The model under review builds one solid part; all positions refer to its coordinate system, in mm. Face numbers are marked on the shaded views. Coordinates: 2 decimals unless noted, no trailing zeros. Write each loop counter-clockwise with the first axis right and the second up, starting at its lowest first coordinate (ties: lowest second). Pieces come first, ordered by that corner, then holes. Notation, with made-up numbers: (40.5, 55) - (90.5, 55) arc R7 ccw to (90.5, 62) - close; hole circle Ø3 at (58.5, 31). An arc over 180 degrees is marked (long way). Put each result on its own line as item: value.
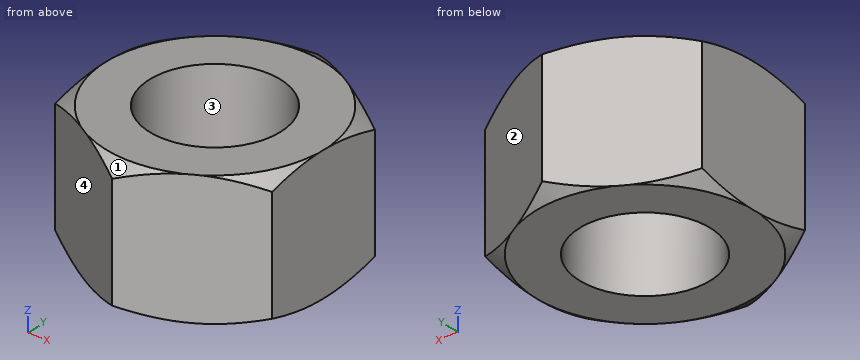
from build123d import *

# Parameters (mm, degrees)
BASENUT_START = -6.1
BASENUTSKE_R  = 3
BASENUT_DEPTH = 6.1


with BuildPart() as part:
    # BaseNutSke → BaseNut (new body)
    with BuildSketch(Plane.XY.offset(BASENUT_START)):
        Polygon((5, 2.886751346), (5, -2.886751346), (0, -5.773502692), (-5, -2.886751346), (-5, 2.886751346), (0, 5.773502692), align=None)
        Circle(BASENUTSKE_R, mode=Mode.SUBTRACT)
    extrude(amount=BASENUT_DEPTH)

    # Sketch3 → Double-Chamfer (revolve, cut)
    with BuildSketch(Plane(origin=(0, 0, 0), x_dir=(0, 0, -1), z_dir=(1, 0, 0))):
        Polygon((6.1, 5), (5.653418013, 5.773502692), (5.653418013, 15.773502692), (16.1, 15.773502692), (16.1, 5), align=None)
        Polygon((0.446581987, 15.773502692), (-10, 15.773502692), (-10, 5), (0, 5), (0.446581987, 5.773502692), align=None)
    revolve(axis=Axis((0, 0, 0), (0, 0, -1)), mode=Mode.SUBTRACT)

    # Sketch5 → EndChamfer (revolve, cut)
    with BuildSketch(Plane(origin=(0, 0, 0), x_dir=(0, 0, -1), z_dir=(1, 0, 0))):
        Polygon((6.0746, 3), (5.689485854, 2.45), (6.1254, 2.45), (6.1254, 3), align=None)
        Polygon((-0.0508, 3), (0, 3), (0.385114146, 2.45), (-0.0508, 2.45), align=None)
    revolve(axis=Axis((0, 0, -25.037505729), (0, 0, -1)), mode=Mode.SUBTRACT)


solid = part.part
1. For pin 1 Ø1 at (x, z) = (2, -1.5) entering from -Y; pin 2 Ø1.5 at (x, z) = (2, -1.5) entering from -Y, all flat-tipped, find the tip position at first contact; note any pin that passes through.
Determined:
pin 1: stops at y = -4.91
pin 2: stops at y = -5.05
2. The part is to be moulded in two halves that separate along X. For the marked faces 1, 2, 3 and 4, say which applies: +X half, -X half, draft (parallel to the pull), parting line (faces both ways), or undercut.
Determined:
face 1: parting line
face 2: +X half
face 3: undercut
face 4: -X half
3. Consider section A-A on z = -3.5. State the section outline as (x, y) points, plus the area to 3 significant figures.
Determined:
outline: (-5, -2.89) - (0, -5.77) - (5, -2.89) - (5, 2.89) - (0, 5.77) - (-5, 2.89) - close; hole circle Ø6 at (0, 0)
area: 58.3 mm^2
4. To check wall thickness, follow probe 1 along X at (y, z) = (0, -3.75); probe 2 along X at (y, z) = (2.75, -1); probe 3 along Y at (x, z) = (1, -3.25). State the ranges of each line that lie inside material, in increasing order.
Determined:
probe 1: x = -5 to -3, 3 to 5
probe 2: x = -5 to -1.2, 1.2 to 5
probe 3: y = -5.2 to -2.83, 2.83 to 5.2
